Verification items for the finished model (mm, model axes). A direction names the side the tool comes from. Round coordinates to 2 decimals unless told otherwise and drop trailing zeros. Loops run counter-clockwise (first coordinate to the right, second up) from the corner with the lowest first, then second, coordinate; pieces in that order, holes last. Notation, with made-up numbers: M 63,75.5 L 76,75.5 A23 cw 76,100.5 Z; hole C 56,4.5 d10. An arc over 180 degrees is marked long. One line per item, written item: value.
from build123d import *

# Parameters (mm, degrees)
SKETCH1_R           = 5.5
SKETCH1_R_2         = 1.3
BOSS_EXTRUDE1_DEPTH = 15
CUT_EXTRUDE1_START  = -2.925993492
CUT_EXTRUDE1_DEPTH  = 2.925993492


with BuildPart() as part:
    # Sketch1 → Boss-Extrude1 (new body)
    with BuildSketch(Plane.XY):
        Circle(SKETCH1_R)
        Circle(SKETCH1_R_2, mode=Mode.SUBTRACT)
    extrude(amount=BOSS_EXTRUDE1_DEPTH)

    # Sketch3 → Cut-Revolve1 (revolve, cut)
    with BuildSketch(Plane(origin=(0, 0, 0), x_dir=(1, 0, 0), z_dir=(0, 1, 0)), mode=Mode.PRIVATE) as cut_revolve1_sk:
        with BuildLine():
            Line((-2.1, -5), (-5.5, -10.001935684))
            Line((-5.5, -10.001935684), (-5.5, 0))
            Line((-5.5, 0), (-2.1, 0))
            ThreePointArc((-2.1, 0), (-2.307106781, -0.5), (-2.1, -1))
            Line((-2.1, -1), (-2.1, -5))
        make_face()
        with BuildLine():
            Line((-2.1, -15), (-4, -15))
            Line((-4, -15), (-4, -10))
            Line((-4, -10), (-2.1, -10))
            Line((-2.1, -10), (-2.1, -14))
            ThreePointArc((-2.1, -14), (-2.307106781, -14.5), (-2.1, -15))
        make_face()
        with BuildLine():
            Line((-5.5, -15), (-5, -15))
            ThreePointArc((-5, -15), (-5.248310238, -14.268501627), (-5, -13.537003254))
            Line((-5, -13.537003254), (-5, -12.074006508))
            Line((-5, -12.074006508), (-5.5, -12.074006508))
            Line((-5.5, -12.074006508), (-5.5, -15))
        make_face()
    revolve(cut_revolve1_sk.sketch.rotate(Axis((0, 0, 15), (0, 0, -1)), 180), axis=Axis((0, 0, 15), (0, 0, -1)), mode=Mode.SUBTRACT)

    # Sketch4 → Cut-Extrude1 (cut)
    with BuildSketch(Plane.XY.offset(15).offset(CUT_EXTRUDE1_START)):
        with BuildLine():
            Line((0, -4), (0, -5.5))
            ThreePointArc((0, -5.5), (-0.493930774, -5.477776227), (-0.98386991, -5.411284506))
            Line((-0.98386991, -5.411284506), (-0.715541753, -3.93547964))
            ThreePointArc((-0.715541753, -3.93547964), (-0.359222381, -3.983837256), (0, -4))
        make_face()
        with BuildLine():
            Line((-4, 0), (-5.5, 0))
            ThreePointArc((-5.5, 0), (-5.477776227, 0.493930774), (-5.411284506, 0.98386991))
            Line((-5.411284506, 0.98386991), (-3.93547964, 0.715541753))
            ThreePointArc((-3.93547964, 0.715541753), (-3.983837256, 0.359222381), (-4, 0))
        make_face()
        with BuildLine():
            Line((0, 4), (0, 5.5))
            ThreePointArc((0, 5.5), (0.493930774, 5.477776227), (0.98386991, 5.411284506))
            Line((0.98386991, 5.411284506), (0.715541753, 3.93547964))
            ThreePointArc((0.715541753, 3.93547964), (0.359222381, 3.983837256), (0, 4))
        make_face()
        with BuildLine():
            Line((4, 0), (5.5, 0))
            ThreePointArc((5.5, 0), (5.477776227, -0.493930774), (5.411284506, -0.98386991))
            Line((5.411284506, -0.98386991), (3.93547964, -0.715541753))
            ThreePointArc((3.93547964, -0.715541753), (3.983837256, -0.359222381), (4, 0))
        make_face()
    extrude(amount=CUT_EXTRUDE1_DEPTH, mode=Mode.SUBTRACT)


solid = part.part
(1) Mould release check, pull along X, two halves, no side actions. Record for faces 1 (the face through (3, -3, 15)), 2 (the face through (2.003, -0.631, 3.028)), 3 (the face through (0.8, 4.4, 13.5)), 4 (the face through (1.846, 3.549, 12.465)): +X half, -X half, draft (parallel to the pull), parting line (faces both ways), or undercut.
Completed:
face 1: draft
face 2: parting line
face 3: undercut
face 4: undercut
(2) Sectioned sample at B-B on z = 10.75. Enter the section's corners in (x, y), and give its area (3 significant figures).
Completed:
outline: C 0,0 d11; C 0,0 d4.2; hole C 0,0 d8; hole C 0,0 d2.6
area: 53.3 mm^2
(3) Sectioned sample at D-D on z = 8.5. Enter the section's corners in (x, y).
Completed:
outline: C 0,0 d8.96; hole C 0,0 d2.6
(4) Depth check by flat-ended pin: pin 1 Ø0.6 at (y, z) = (4.5, 13.5) entering from +X; pin 2 Ø2 at (x, y) = (3.5, 0) entering from -Z; pin 3 Ø1 at (y, z) = (-4.5, 14.5) entering from -X. Enter the tip coordinate at first touch or a pass-through.
Completed:
pin 1: stops at x = 2.79
pin 2: stops at z = 5.59
pin 3: stops at x = -3.38
(5) Tool access check on faces 5 (the face through (0, 4.5, 13.5)), 6 (the face through (4, 3, 13)), 7 (the face through (0, -4.5, 13.5)), 8 (the face through (4.5, 0, 13.5)), 9 (the face through (-4.4, 0.8, 13.5)). Record the directions out of +Z, -Z, +X, -X, +Y, -Y that give a thin tool (end or side, any length) a straight path to the whole face; none if there is none.
Completed:
face 5: +Z, +Y
face 6: +X, +Y
face 7: +Z, -Y
face 8: +Z, +X
face 9: +Z, -X
(6) Thickness scan on L1, parallel to Y at x = 1.5, z = 13; L2, parallel to Y at x = 0, z = 4.75; L3, parallel to Y at x = -0.25, z = 10.5. Record the ranges inside material, lowest first. Write a range as from..to.
Completed:
L1: y = -4.77..-3.71, -1.47..1.47, 3.71..4.77
L2: y = -2.1..-1.3, 1.3..2.1
L3: y = -5.49..-3.99, -2.09..-1.28, 1.28..2.09, 3.99..5.49
(7) Sectioned sample at A-A on z = 12.75. Enter the section's corners in (x, y).
Completed:
outline: M -5,0 A5 ccw -0.89,-4.92 L -0.72,-3.94 A4 cw -4,0 Z; M -4.92,0.89 L -3.94,0.72 A4 cw 0,4 L 0,5 A5 ccw Z; C 0,0 d4.2; M 0,-5 A5 ccw 4.92,-0.89 L 3.94,-0.72 A4 cw 0,-4 Z; M 0.72,3.94 A4 cw 4,0 L 5,0 A5 ccw 0.89,4.92 Z; hole C 0,0 d2.6
(8) Sectioned sample at C-C on z = 3.75. Enter the section's corners in (x, y), and give its area (3 significant figures).
Completed:
outline: C 0,0 d4.2; hole C 0,0 d2.6
area: 8.55 mm^2
